Geometry: final body of the model. Coordinates: model frame, mm. A direction names the side the tool comes from. Give positions to 0.01 mm unless a question says otherwise; leave off trailing zeros. Order: outer loops, then holes, each group sorted by start corner. A loop starts at its lowest first (then second) coordinate and runs counter-clockwise, first axis right, second up. Notation, with made-up numbers: (59.5, 7) - (104.5, 7) arc R18 cw to (104.5, 32) - close; hole circle Ø10 at (37.5, 86). An arc over 180 degrees is marked (long way). One line per item, written item: value.
```python
from build123d import *

# Parameters (mm, degrees)
BOSS_EXTRUDE1_DEPTH = 14
SKETCH2_R           = 3
BOSS_EXTRUDE2_DEPTH = 3
CUT_EXTRUDE1_DEPTH  = 8
CUT_EXTRUDE2_START  = -6
SKETCH4_R           = 1.5
CUT_EXTRUDE2_DEPTH  = 6


with BuildPart() as part:
    # Sketch1 → Boss-Extrude1 (new body)
    with BuildSketch(Plane(origin=(0, 0, 0), x_dir=(1, 0, 0), z_dir=(0, 1, 0))):
        with BuildLine():
            Line((-6.5, 15.165750888), (-6.5, 10))
            ThreePointArc((-6.5, 10), (0, 3.5), (6.5, 10))
            Line((6.5, 10), (6.5, 15.165750888))
            ThreePointArc((6.5, 15.165750888), (16.5, 0), (6.5, -15.165750888))
            Line((6.5, -15.165750888), (6.5, -10))
            ThreePointArc((6.5, -10), (0, -3.5), (-6.5, -10))
            Line((-6.5, -10), (-6.5, -15.165750888))
            ThreePointArc((-6.5, -15.165750888), (-16.5, 0), (-6.5, 15.165750888))
        make_face()
    extrude(amount=BOSS_EXTRUDE1_DEPTH)

    # Sketch2 → Boss-Extrude2 (add)
    with BuildSketch(Plane.XZ):
        with Locations(Location((0, 0, 0), (0, 0, 270))):
            Circle(SKETCH2_R)
    extrude(amount=BOSS_EXTRUDE2_DEPTH)

    # Sketch3 → Cut-Extrude1 (cut)
    with BuildSketch(Plane.XZ.offset(3)):
        with BuildLine():
            Line((0.997797575, 1.12), (0.997797575, -1.12))
            ThreePointArc((0.997797575, -1.12), (-1.5, 0), (0.997797575, 1.12))
        make_face()
    extrude(amount=-CUT_EXTRUDE1_DEPTH, mode=Mode.SUBTRACT)

    # Sketch4 → Cut-Extrude2 (cut)
    with BuildSketch(Plane(origin=(0, 14, 0), x_dir=(1, 0, 0), z_dir=(0, 1, 0)).offset(CUT_EXTRUDE2_START)):
        with Locations(Location((0, 0, 0), (0, 0, 270))):
            Circle(SKETCH4_R)
    extrude(amount=CUT_EXTRUDE2_DEPTH, mode=Mode.SUBTRACT)


solid = part.part
```
1) Section B-B, the plane z = -7.5. Return loops of the section in (x, y).
Answers below:
outline: (-14.7, 0) - (-6, 0) - (-6, 14) - (-14.7, 14) - close; (6, 0) - (14.7, 0) - (14.7, 14) - (6, 14) - close
2) Section A-A, the plane y = 11.5. Return loops of the section in (x, z), then the cut area to 3 significant figures.
Answers below:
outline: (-6.5, -15.17) - (-6.5, -10) arc R6.5 cw to (6.5, -10) - (6.5, -15.17) arc R16.5 ccw to (6.5, 15.17) - (6.5, 10) arc R6.5 cw to (-6.5, 10) - (-6.5, 15.17) arc R16.5 ccw to start; hole circle Ø3 at (0, 0)
area: 558 mm^2
3) Section D-D, the plane x = 0. Return loops of the section in (y, z).
Answers below:
outline: (-3, -3) - (0, -3) - (0, -3.5) - (14, -3.5) - (14, -1.5) - (8, -1.5) - (8, 1.5) - (14, 1.5) - (14, 3.5) - (0, 3.5) - (0, 3) - (-3, 3) - (-3, 1.5) - (5, 1.5) - (5, -1.5) - (-3, -1.5) - close
4) Material intervals for line 1 along Y through (x, z) = (-12, 10); line 2 along X through (y, z) = (4.25, -0.5); line 3 along X through (y, z) = (7.5, 12), sorted ascending.
Answers below:
line 1: 0 to 14
line 2: -16.49 to -1.41, 1 to 16.49
line 3: -11.32 to -6.5, 6.5 to 11.32
5) Section C-C, the plane z = 0. Return loops of the section in (x, y), then the cut area to 3 significant figures.
Answers below:
outline: (-16.5, 0) - (-3, 0) - (-3, -3) - (-1.5, -3) - (-1.5, 5) - (1, 5) - (1, -3) - (3, -3) - (3, 0) - (16.5, 0) - (16.5, 14) - (1.5, 14) - (1.5, 8) - (-1.5, 8) - (-1.5, 14) - (-16.5, 14) - close
area: 442 mm^2
6) Mould query, pull axis X, two halves, no side actions, for faces 1 (the face through (0.9, -1.48, -2.86)), 2 (the face through (-16.498, 6.902, 0.269)), 3 (the face through (1.4, -3, 0)), 4 (the face through (6.5, 7, 13)). Classes: released by +X, released by -X, zero draft, split by the parting line, or undercut.
Answers below:
face 1: split by the parting line
face 2: released by -X
face 3: zero draft
face 4: undercut
7) First-contact query: pin 1 (1 mm diameter, centred on x = 13, y = 3.5, fed in from -Z); pin 2 (0.7 mm diameter, centred on y = 2, z = 0.5, fed in from -X); pin 3 (4 mm diameter, centred on y = 2, z = -6, fed in from +X). Flat tips, straight axial feed; report the tip coordinate or a pass-through.
Answers below:
pin 1: z = -10.77
pin 2: x = -16.5
pin 3: x = 16.01
8) Set-up query: faces 5 (the face through (-6.5, 7, 13)), 6 (the face through (0, 14, 3)), 7 (the face through (0, 5, 0)), 8 (the face through (6.5, 7, -13)), 9 (the face through (0, 8, 0)). Return all of +Z, -Z, +X, -X, +Y, -Y with unobstructed straight access to the full face (end or side cutting, diameter ignored); none if empty.
Answers below:
face 5: +Z, +Y, -Y
face 6: +Z, -Z, +X, -X, +Y
face 7: -Y
face 8: -Z, +Y, -Y
face 9: +Y
